CAD build for the part. Positions are in the model's coordinates, mm. Round coordinates to 2 decimals unless told otherwise and drop trailing zeros. Write each loop counter-clockwise with the first axis right and the second up, starting at its lowest first coordinate (ties: lowest second). Pieces come first, ordered by that corner, then holes. Notation, with made-up numbers: (79, 76.25) - (137, 76.25) arc R21 cw to (137, 113.25) - close; hole circle Ø1 at (60, 70). An arc over 180 degrees is marked (long way). Put each result on its own line as item: value. Start each with the question number.
Item 1: Cut at B-B (x = -49). Give the cut face in (y, z), and give its area (3 significant figures).
Item 2: Drill centre lines: line 1 (X direction, y = -1.25, z = 7); line 2 (X direction, y = -0.65, z = 8.5); line 3 (Z direction, x = -31, y = -2.05). Where is each one in solid material? Low to high. Write a range as from..to.
Item 3: Cut at D-D (x = -17). Give the cut face in (y, z), and give its area (3 significant figures).
Item 4: Cut at A-A (z = 12). Give the cut face in (x, y), and give its area (3 significant figures).
Item 5: Cut at C-C (y = -0.9). Give the cut face in (x, z).
Item 6: Pin check, flat tip, straight feed: pin 1 Ø7.5 at (x, z) = (-33.57, 43.5) entering from -Y. Stop position of the tip, or through.
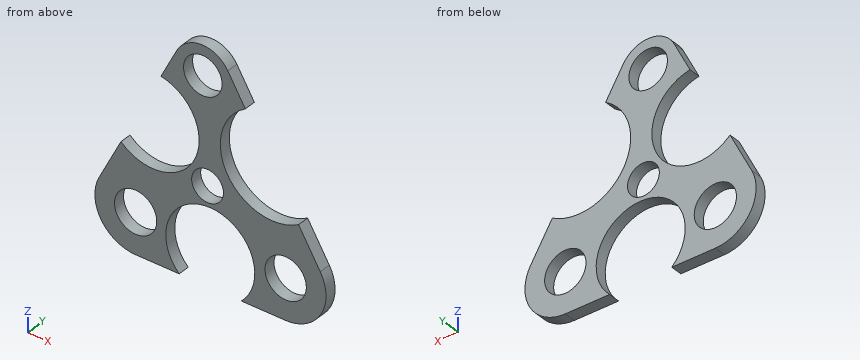
```python
from build123d import *

# Parameters (mm, degrees)
F1_DEPTH = 2.54
F2_R     = 3.465716
F3_DEPTH = 25.4
F4_R     = 4.599805
F4_R_2   = 4.505761
F5_DEPTH = 25.4
F6_R     = 4.197487
F7_DEPTH = 25.4


with BuildPart() as f1:
    # F0 (on Front) → F1 (new body)
    with BuildSketch(Plane.XZ):
        with BuildLine():
            ThreePointArc((-15.541226, 0), (-7.891157, 4.462448), (-8.00983, 13.318121))
            Line((-8.00983, 13.318121), (-12.724322, 21.157009))
            ThreePointArc((-12.724322, 21.157009), (-28.161806, 24.999227), (-24.319587, 40.436711))
            Line((-24.319587, 40.436711), (-28.128936, 46.770598))
            ThreePointArc((-28.128936, 46.770598), (-33.807833, 49.843423), (-39.241434, 46.355143))
            Line((-39.241434, 46.355143), (-42.67387, 39.542808))
            ThreePointArc((-42.67387, 39.542808), (-35.450995, 25.066238), (-51.383585, 22.256688))
            Line((-51.383585, 22.256688), (-56.11723, 12.861851))
            ThreePointArc((-56.11723, 12.861851), (-55.748343, 4.218604), (-48.195517, 0))
            Line((-48.195517, 0), (-38.709875, 0))
            ThreePointArc((-38.709875, 0), (-31.946439, 16.630052), (-25.183003, 0))
            Line((-25.183003, 0), (-15.541226, 0))
        make_face()
    extrude(amount=F1_DEPTH)

    # F2 (on face) → F3 (cut)
    with BuildSketch(Plane.XZ.offset(2.54)):
        with Locations((-32.539293, 20.90759)):
            Circle(F2_R)
    extrude(amount=-F3_DEPTH, mode=Mode.SUBTRACT)

    # F4 (on face) → F5 (cut)
    with BuildSketch(Plane.XZ.offset(2.54)):
        with Locations((-48.195517, 8.870448)):
            Circle(F4_R)
        with Locations((-15.541226, 8.788562)):
            Circle(F4_R_2)
    extrude(amount=-F5_DEPTH, mode=Mode.SUBTRACT)

    # F6 (on face) → F7 (cut)
    with BuildSketch(Plane.XZ.offset(2.54)):
        with Locations((-33.570595, 43.497856)):
            Circle(F6_R)
    extrude(amount=-F7_DEPTH, mode=Mode.SUBTRACT)


solid = f1.part
```
Output values:
1. outline: (-2.54, 0.04) - (0, 0.04) - (0, 4.34) - (-2.54, 4.34) - close; (-2.54, 13.4) - (0, 13.4) - (0, 20.59) - (-2.54, 20.59) - close
1. area: 29.2 mm2
2. line 1: -56.87..-52.4, -43.99..-41.64, -22.26..-19.68, -11.41..-6.94
2. line 2: -57.06..-52.78, -43.61..-41.51, -22.38..-20.04, -11.04..-6.76
2. line 3: 16.58..17.8, 24.01..40.18, 46.82..49.3
3. outline: (-2.54, 0) - (0, 0) - (0, 4.53) - (-2.54, 4.53) - close; (-2.54, 13.05) - (0, 13.05) - (0, 19.65) - (-2.54, 19.65) - close
3. area: 28.3 mm2
4. outline: (-56.5, -2.54) - (-51.57, -2.54) - (-51.57, 0) - (-56.5, 0) - close; (-44.82, -2.54) - (-40.21, -2.54) - (-40.21, 0) - (-44.82, 0) - close; (-23.68, -2.54) - (-18.7, -2.54) - (-18.7, 0) - (-23.68, 0) - close; (-12.38, -2.54) - (-7.36, -2.54) - (-7.36, 0) - (-12.38, 0) - close
4. area: 49.6 mm2
5. outline: (-56.12, 12.86) arc R8.87 ccw to (-48.2, 0) - (-38.71, 0) arc R9.69 cw (long way) to (-25.18, 0) - (-15.54, 0) arc R8.79 ccw to (-8.01, 13.32) - (-12.72, 21.16) arc R11.25 cw to (-24.32, 40.44) - (-28.13, 46.77) arc R6.35 ccw to (-39.24, 46.36) - (-42.67, 39.54) arc R10.09 cw (long way) to (-51.38, 22.26) - close; hole circle Ø9.2 at (-48.2, 8.87); hole circle Ø8.39 at (-33.57, 43.5); hole circle Ø6.93 at (-32.54, 20.91); hole circle Ø9.01 at (-15.54, 8.79)
6. pin 1: through
